Part model, mm, in its own coordinate system. Round coordinates to 2 decimals unless told otherwise and drop trailing zeros. Order: outer loops, then holes, each group sorted by start corner. A loop starts at its lowest first (then second) coordinate and runs counter-clockwise, first axis right, second up. Notation, with made-up numbers: (-33.75, 45.25) -> (3.25, 45.25) arc R19 cw to (3.25, 65.25) -> close; hole circle Ø7 at (13, 83). An arc over 180 degrees is marked (long way). Answer as a JSON object with one key per item and string values. Group by question number.
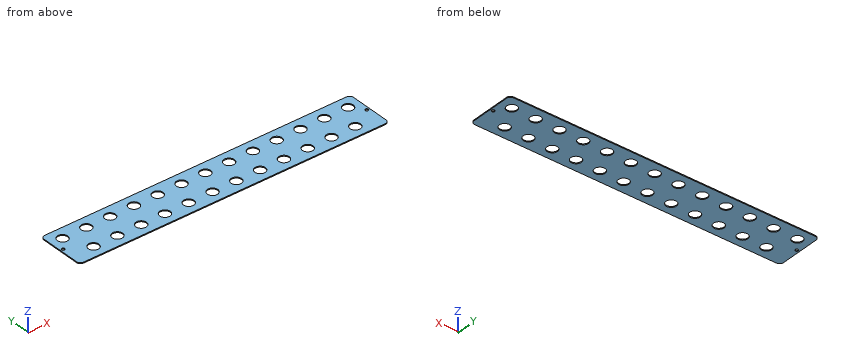
```python
from build123d import *

# Parameters (mm, degrees)
BOSS_EXTRUDE1_DEPTH      = 2
SKETCH2_R                = 3
CUT_EXTRUDE2_DEPTH       = 10
LPATTERN1_COUNT          = 13
LPATTERN1_PITCH          = 50
LPATTERN2_COUNT          = 2
LPATTERN2_PITCH          = 50
LPATTERN2_COUNT_DIR2     = 2
LPATTERN2_PITCH_DIR2     = 25.5
M6_CLEARANCE_HOLE2_D     = 6.6
M6_CLEARANCE_HOLE2_DEPTH = 6
M6_CLEARANCE_HOLE2_TIP   = 1.982840043


with BuildPart() as part:
    # Sketch1 → Boss-Extrude1 (new body)
    with BuildSketch(Plane.XY):
        with BuildLine():
            Line((-316.901308233, -50), (316.901308233, -50))
            ThreePointArc((316.901308233, -50), (322.6279481, -47.6279481), (325, -41.901308233))
            Line((325, -41.901308233), (325, 41.901308233))
            ThreePointArc((325, 41.901308233), (322.6279481, 47.6279481), (316.901308233, 50))
            Line((316.901308233, 50), (-316.901308233, 50))
            ThreePointArc((-316.901308233, 50), (-322.6279481, 47.6279481), (-325, 41.901308233))
            Line((-325, 41.901308233), (-325, -41.901308233))
            ThreePointArc((-325, -41.901308233), (-322.6279481, -47.6279481), (-316.901308233, -50))
        make_face()
    extrude(amount=BOSS_EXTRUDE1_DEPTH)

    # Sketch2 → Cut-Extrude2 (cut)
    with BuildSketch(Plane.XY.offset(2)):
        with Locations((300, 25)):
            Circle(SKETCH2_R)
        with Locations((-319, 0)):
            Circle(SKETCH2_R)
        with Locations((319, 0)):
            Circle(SKETCH2_R)
    extrude(amount=-CUT_EXTRUDE2_DEPTH, mode=Mode.SUBTRACT)

    # Sketch5 → M20 Clearance Hole2 (revolve, cut)
    with BuildSketch(Plane(origin=(300, 25, 2), x_dir=(0, -1, 0), z_dir=(1, 0, 0))):
        Polygon((0, 0), (0, 12.609466809), (11, 6), (11, 0), align=None)
    m20_clearance_hole2 = revolve(axis=Axis((300, 25, 8.35), (0, 0, -1)), mode=Mode.SUBTRACT)

    # LPattern1: M20 Clearance Hole2 ×13
    with Locations(*[(-i * LPATTERN1_PITCH, 0, 0) for i in range(1, LPATTERN1_COUNT)]):
        add(m20_clearance_hole2, mode=Mode.SUBTRACT)

    # LPattern2: M20 Clearance Hole2 2 × 2, 2 skipped
    with Locations(*[(-j * LPATTERN2_PITCH_DIR2, -i * LPATTERN2_PITCH, 0) for i in range(LPATTERN2_COUNT) for j in range(LPATTERN2_COUNT_DIR2) if (i, j) not in ((0, 0), (0, 1), (1, 0))]):
        add(m20_clearance_hole2, mode=Mode.SUBTRACT)

    # LPattern3 copy 1 sketch → LPattern3 copy 1 (revolve, cut)
    with BuildSketch(Plane(origin=(224.5, -25, 2), x_dir=(0, -1, 0), z_dir=(1, 0, 0))):
        Polygon((0, 0), (0, 12.609466809), (11, 6), (11, 0), align=None)
    revolve(axis=Axis((224.5, -25, 8.35), (0, 0, -1)), mode=Mode.SUBTRACT)

    # LPattern3 copy 2 sketch → LPattern3 copy 2 (revolve, cut)
    with BuildSketch(Plane(origin=(174.5, -25, 2), x_dir=(0, -1, 0), z_dir=(1, 0, 0))):
        Polygon((0, 0), (0, 12.609466809), (11, 6), (11, 0), align=None)
    revolve(axis=Axis((174.5, -25, 8.35), (0, 0, -1)), mode=Mode.SUBTRACT)

    # LPattern3 copy 3 sketch → LPattern3 copy 3 (revolve, cut)
    with BuildSketch(Plane(origin=(124.5, -25, 2), x_dir=(0, -1, 0), z_dir=(1, 0, 0))):
        Polygon((0, 0), (0, 12.609466809), (11, 6), (11, 0), align=None)
    revolve(axis=Axis((124.5, -25, 8.35), (0, 0, -1)), mode=Mode.SUBTRACT)

    # LPattern3 copy 4 sketch → LPattern3 copy 4 (revolve, cut)
    with BuildSketch(Plane(origin=(74.5, -25, 2), x_dir=(0, -1, 0), z_dir=(1, 0, 0))):
        Polygon((0, 0), (0, 12.609466809), (11, 6), (11, 0), align=None)
    revolve(axis=Axis((74.5, -25, 8.35), (0, 0, -1)), mode=Mode.SUBTRACT)

    # LPattern3 copy 5 sketch → LPattern3 copy 5 (revolve, cut)
    with BuildSketch(Plane(origin=(24.5, -25, 2), x_dir=(0, -1, 0), z_dir=(1, 0, 0))):
        Polygon((0, 0), (0, 12.609466809), (11, 6), (11, 0), align=None)
    revolve(axis=Axis((24.5, -25, 8.35), (0, 0, -1)), mode=Mode.SUBTRACT)

    # LPattern3 copy 6 sketch → LPattern3 copy 6 (revolve, cut)
    with BuildSketch(Plane(origin=(-25.5, -25, 2), x_dir=(0, -1, 0), z_dir=(1, 0, 0))):
        Polygon((0, 0), (0, 12.609466809), (11, 6), (11, 0), align=None)
    revolve(axis=Axis((-25.5, -25, 8.35), (0, 0, -1)), mode=Mode.SUBTRACT)

    # LPattern3 copy 7 sketch → LPattern3 copy 7 (revolve, cut)
    with BuildSketch(Plane(origin=(-75.5, -25, 2), x_dir=(0, -1, 0), z_dir=(1, 0, 0))):
        Polygon((0, 0), (0, 12.609466809), (11, 6), (11, 0), align=None)
    revolve(axis=Axis((-75.5, -25, 8.35), (0, 0, -1)), mode=Mode.SUBTRACT)

    # LPattern3 copy 8 sketch → LPattern3 copy 8 (revolve, cut)
    with BuildSketch(Plane(origin=(-125.5, -25, 2), x_dir=(0, -1, 0), z_dir=(1, 0, 0))):
        Polygon((0, 0), (0, 12.609466809), (11, 6), (11, 0), align=None)
    revolve(axis=Axis((-125.5, -25, 8.35), (0, 0, -1)), mode=Mode.SUBTRACT)

    # LPattern3 copy 9 sketch → LPattern3 copy 9 (revolve, cut)
    with BuildSketch(Plane(origin=(-175.5, -25, 2), x_dir=(0, -1, 0), z_dir=(1, 0, 0))):
        Polygon((0, 0), (0, 12.609466809), (11, 6), (11, 0), align=None)
    revolve(axis=Axis((-175.5, -25, 8.35), (0, 0, -1)), mode=Mode.SUBTRACT)

    # LPattern3 copy 10 sketch → LPattern3 copy 10 (revolve, cut)
    with BuildSketch(Plane(origin=(-225.5, -25, 2), x_dir=(0, -1, 0), z_dir=(1, 0, 0))):
        Polygon((0, 0), (0, 12.609466809), (11, 6), (11, 0), align=None)
    revolve(axis=Axis((-225.5, -25, 8.35), (0, 0, -1)), mode=Mode.SUBTRACT)

    # LPattern3 copy 11 sketch → LPattern3 copy 11 (revolve, cut)
    with BuildSketch(Plane(origin=(-275.5, -25, 2), x_dir=(0, -1, 0), z_dir=(1, 0, 0))):
        Polygon((0, 0), (0, 12.609466809), (11, 6), (11, 0), align=None)
    revolve(axis=Axis((-275.5, -25, 8.35), (0, 0, -1)), mode=Mode.SUBTRACT)

    # LPattern3 copy 12 sketch → LPattern3 copy 12 (revolve, cut)
    with BuildSketch(Plane(origin=(250, 25, 2), x_dir=(0, -1, 0), z_dir=(1, 0, 0))):
        Polygon((0, 0), (0, 12.609466809), (11, 6), (11, 0), align=None)
    revolve(axis=Axis((250, 25, 8.35), (0, 0, -1)), mode=Mode.SUBTRACT)

    # LPattern3 copy 13 sketch → LPattern3 copy 13 (revolve, cut)
    with BuildSketch(Plane(origin=(200, 25, 2), x_dir=(0, -1, 0), z_dir=(1, 0, 0))):
        Polygon((0, 0), (0, 12.609466809), (11, 6), (11, 0), align=None)
    revolve(axis=Axis((200, 25, 8.35), (0, 0, -1)), mode=Mode.SUBTRACT)

    # LPattern3 copy 14 sketch → LPattern3 copy 14 (revolve, cut)
    with BuildSketch(Plane(origin=(150, 25, 2), x_dir=(0, -1, 0), z_dir=(1, 0, 0))):
        Polygon((0, 0), (0, 12.609466809), (11, 6), (11, 0), align=None)
    revolve(axis=Axis((150, 25, 8.35), (0, 0, -1)), mode=Mode.SUBTRACT)

    # LPattern3 copy 15 sketch → LPattern3 copy 15 (revolve, cut)
    with BuildSketch(Plane(origin=(100, 25, 2), x_dir=(0, -1, 0), z_dir=(1, 0, 0))):
        Polygon((0, 0), (0, 12.609466809), (11, 6), (11, 0), align=None)
    revolve(axis=Axis((100, 25, 8.35), (0, 0, -1)), mode=Mode.SUBTRACT)

    # LPattern3 copy 16 sketch → LPattern3 copy 16 (revolve, cut)
    with BuildSketch(Plane(origin=(50, 25, 2), x_dir=(0, -1, 0), z_dir=(1, 0, 0))):
        Polygon((0, 0), (0, 12.609466809), (11, 6), (11, 0), align=None)
    revolve(axis=Axis((50, 25, 8.35), (0, 0, -1)), mode=Mode.SUBTRACT)

    # LPattern3 copy 17 sketch → LPattern3 copy 17 (revolve, cut)
    with BuildSketch(Plane(origin=(0, 25, 2), x_dir=(0, -1, 0), z_dir=(1, 0, 0))):
        Polygon((0, 0), (0, 12.609466809), (11, 6), (11, 0), align=None)
    revolve(axis=Axis((0, 25, 8.35), (0, 0, -1)), mode=Mode.SUBTRACT)

    # LPattern3 copy 18 sketch → LPattern3 copy 18 (revolve, cut)
    with BuildSketch(Plane(origin=(-50, 25, 2), x_dir=(0, -1, 0), z_dir=(1, 0, 0))):
        Polygon((0, 0), (0, 12.609466809), (11, 6), (11, 0), align=None)
    revolve(axis=Axis((-50, 25, 8.35), (0, 0, -1)), mode=Mode.SUBTRACT)

    # LPattern3 copy 19 sketch → LPattern3 copy 19 (revolve, cut)
    with BuildSketch(Plane(origin=(-100, 25, 2), x_dir=(0, -1, 0), z_dir=(1, 0, 0))):
        Polygon((0, 0), (0, 12.609466809), (11, 6), (11, 0), align=None)
    revolve(axis=Axis((-100, 25, 8.35), (0, 0, -1)), mode=Mode.SUBTRACT)

    # LPattern3 copy 20 sketch → LPattern3 copy 20 (revolve, cut)
    with BuildSketch(Plane(origin=(-150, 25, 2), x_dir=(0, -1, 0), z_dir=(1, 0, 0))):
        Polygon((0, 0), (0, 12.609466809), (11, 6), (11, 0), align=None)
    revolve(axis=Axis((-150, 25, 8.35), (0, 0, -1)), mode=Mode.SUBTRACT)

    # LPattern3 copy 21 sketch → LPattern3 copy 21 (revolve, cut)
    with BuildSketch(Plane(origin=(-200, 25, 2), x_dir=(0, -1, 0), z_dir=(1, 0, 0))):
        Polygon((0, 0), (0, 12.609466809), (11, 6), (11, 0), align=None)
    revolve(axis=Axis((-200, 25, 8.35), (0, 0, -1)), mode=Mode.SUBTRACT)

    # LPattern3 copy 22 sketch → LPattern3 copy 22 (revolve, cut)
    with BuildSketch(Plane(origin=(-250, 25, 2), x_dir=(0, -1, 0), z_dir=(1, 0, 0))):
        Polygon((0, 0), (0, 12.609466809), (11, 6), (11, 0), align=None)
    revolve(axis=Axis((-250, 25, 8.35), (0, 0, -1)), mode=Mode.SUBTRACT)

    # M6 Clearance Hole2
    with Locations(Plane(origin=(0, 0, 0), x_dir=(-1, 0, 0), z_dir=(0, 0, -1))):
        with Locations((319, 0), (-319, 0)):
            Hole(M6_CLEARANCE_HOLE2_D / 2, depth=M6_CLEARANCE_HOLE2_DEPTH)
            with Locations((0, 0, -(M6_CLEARANCE_HOLE2_DEPTH + M6_CLEARANCE_HOLE2_TIP / 2))):  # 118° drill point
                Cone(0, M6_CLEARANCE_HOLE2_D / 2, M6_CLEARANCE_HOLE2_TIP, mode=Mode.SUBTRACT)


solid = part.part
```
Q1. Band-saw the part on A-A (x = 274.5). List the corners of the cut face in (y, z), plus the area to 3 significant figures.
Q2. Drop flat-ended pins along their axis: pin 1 Ø13 at (x, y) = (74.5, -25) entering from -Z; pin 2 Ø8.5 at (x, y) = (319, 0) entering from -Z. Give the stop position or say it passes through.
Q3. Band-saw the part on B-B (y = 25). Count the separate pieces of the cut face and the enclosed holes in it, plus the area to 3 significant figures.
Q4. Wall check: line 1 (Y direction, x = 200, z = 1.4); line 2 (Y direction, x = 224.5, z = 0.9). Give the ranges that are in metal, low to high. Write a range as [from, to].
Completed:
{
 "1": {"outline": "(-50, 0) -> (-36, 0) -> (-36, 2) -> (-50, 2) -> close; (-14, 0) -> (50, 0) -> (50, 2) -> (-14, 2) -> close", "area": "156 mm2"},
 "2": {"pin 1": "through", "pin 2": "z = 0"},
 "3": {"separate pieces": "14", "enclosed holes": "0", "area": "728 mm2"},
 "4": {"line 1": "[-50, 14], [36, 50]", "line 2": "[-50, -36], [-14, 50]"}
}
